```python
from build123d import *

# Parameters (mm, degrees)
SKETCH_1_W     = 15
SKETCH_1_H     = 3
SKETCH_2_W     = 3
SKETCH_2_H     = 6.5
SKETCH_3_W     = 3
SKETCH_3_H     = 9
CHAMFER_1_SIZE = 1
FILLET_2_R     = 1.5


with BuildPart() as part:
    # 草图1 → 旋转1 (revolve)
    with BuildSketch(Plane(origin=(0, 0, 0), x_dir=(0, 0, -1), z_dir=(1, 0, 0)), mode=Mode.PRIVATE) as revolve_1_sk:
        with Locations((-7.5, -7.5)):
            Rectangle(SKETCH_1_W, SKETCH_1_H)
        Polygon((-15, -9), (-15, -6), (-15, 0), (-18, 0), (-18, -9), align=None)
    revolve(revolve_1_sk.sketch.rotate(Axis((0, 0, 0), (0, 0, 1)), 180), axis=Axis((0, 0, 0), (0, 0, 1)))

    # 草图2 → 切除-旋转1 (revolve, cut)
    with BuildSketch(Plane(origin=(0, 0, 0), x_dir=(0, 0, -1), z_dir=(1, 0, 0)), mode=Mode.PRIVATE) as cut_revolve_1_sk:
        with Locations((-16.5, -3.25)):
            Rectangle(SKETCH_2_W, SKETCH_2_H)
    revolve(cut_revolve_1_sk.sketch.rotate(Axis((0, 0, 18), (0, 0, -1)), 270), axis=Axis((0, 0, 18), (0, 0, -1)), mode=Mode.SUBTRACT)

    # 草图3 → 切除-旋转2 (revolve, cut)
    with BuildSketch(Plane(origin=(0, 0, 0), x_dir=(0, 0, -1), z_dir=(1, 0, 0)), mode=Mode.PRIVATE) as cut_revolve_2_sk:
        with Locations((-16.5, -4.5)):
            Rectangle(SKETCH_3_W, SKETCH_3_H)
    revolve(cut_revolve_2_sk.sketch.rotate(Axis((0, 0, 18), (0, 0, -1)), 180), axis=Axis((0, 0, 18), (0, 0, -1)), mode=Mode.SUBTRACT)

    # 倒角1
    chamfer_1_edges = [part.edges().sort_by_distance(p)[0] for p in [
        (0, -9, 0),
    ]]
    chamfer(chamfer_1_edges, length=CHAMFER_1_SIZE)

    # 圆角2
    fillet_2_edges = [part.edges().sort_by_distance(p)[0] for p in [
        (0, -6, 0),
    ]]
    fillet(fillet_2_edges, radius=FILLET_2_R)


solid = part.part
```
CAD build for the part. Positions are in the model's coordinates, mm. Round coordinates to 2 decimals unless told otherwise and drop trailing zeros. Order: outer loops, then holes, each group sorted by start corner. A loop starts at its lowest first (then second) coordinate and runs counter-clockwise, first axis right, second up. Notation, with made-up numbers: (56.25, 83) -> (71.25, 83) arc R24 ccw to (71.25, 113) -> close; hole circle Ø2 at (55, -9.75). An arc over 180 degrees is marked (long way). Write item = value, one per line.
(1) Flat gauge pins, fed straight in: P1, Ø4, axis at y = -6.5, z = 11, coming from the +X side; P2, Ø2, axis at y = 1.5, z = 12.5, coming from the +X side; P3, Ø4, axis at y = -7, z = 4.5, coming from the -X side; P4, Ø2, axis at x = 3.5, y = -2.5, coming from the +Z side. Where does each tip first touch, or does it go through?
Answers follow:
P1 = 7.79
P2 = 8.99
P3 = -7.48
P4 = through
(2) Cut at A-A (x = 0). Write the cut outline in (y, z).
Answers follow:
outline = (-9, 1) -> (-8, 0) -> (-7.5, 0) arc R1.5 ccw to (-6, 1.5) -> (-6, 15) -> (-9, 15) -> close; (6, 1.5) arc R1.5 ccw to (7.5, 0) -> (8, 0) -> (9, 1) -> (9, 15) -> (6, 15) -> close
(3) Drill centre lines: L1, parallel to X at y = 0, z = 7.5; L2, parallel to Y at x = -2.75, z = 6.5; L3, parallel to X at y = 1.5, z = 11.5. Where is each one in solid material? Low to high.
Answers follow:
L1 = -9 to -6, 6 to 9
L2 = -8.57 to -5.33, 5.33 to 8.57
L3 = -8.87 to -5.81, 5.81 to 8.87
(4) Pull direction X, two halves, no side cores. Call faces 1 (the cylindrical face through (-1.802, 5.723, 8.156)), 2 (the cylindrical face through (-6.083, -6.633, 7.902)), 3 (the flat face through (-6, 2, 15)): +X half, -X half, draft (parallel to the pull), parting line (faces both ways), or undercut.
Answers follow:
face_1 = undercut
face_2 = parting line
face_3 = draft
(5) Cut at C-C (z = 4.75). Write the cut outline in (x, y), plus the area to 3 significant figures.
Answers follow:
outline = circle Ø18 at (0, 0); hole circle Ø12 at (0, 0)
area = 141 mm²
